```python
from build123d import *

# Parameters (mm, degrees)
CROQUIS1_R              = 1.5
SALIENTE_EXTRUIR1_DEPTH = 9
CROQUIS2_W              = 20
CROQUIS2_H              = 3.5
CORTAR_EXTRUIR1_DEPTH   = 18
REDONDEO1_R             = 3
CORTAR_EXTRUIR2_START   = -50
CORTAR_EXTRUIR2_DEPTH   = 50


# Read off the part's stored shape, not the designer's step: Cortar-Extruir2
with BuildPart() as part:
    # Croquis1 → Saliente-Extruir1 (new body)
    with BuildSketch(Plane(origin=(0, 0, 0), x_dir=(1, 0, 0), z_dir=(0, 1, 0))):
        Polygon((0, 0), (0, 10), (10, 16), (9, 10), (50, 10), (50, 0), align=None)
        with Locations(Location((25, 6, 0), (0, 0, 270))):
            Circle(CROQUIS1_R, mode=Mode.SUBTRACT)
    extrude(amount=SALIENTE_EXTRUIR1_DEPTH)

    # Croquis2 → Cortar-Extruir1 (cut)
    with BuildSketch(Plane(origin=(0, 9, 0), x_dir=(1, 0, 0), z_dir=(0, 1, 0))):
        with Locations((40, 8.25)):
            Rectangle(CROQUIS2_W, CROQUIS2_H)
    extrude(amount=-CORTAR_EXTRUIR1_DEPTH, mode=Mode.SUBTRACT)

    # Redondeo1
    redondeo1_edges = [part.edges().sort_by_distance(p)[0] for p in [
        (0, 4.5, -10),
        (30, 4.5, -10),
        (50, 4.5, -6.5),
    ]]
    fillet(redondeo1_edges, radius=REDONDEO1_R)

    # Cortar-Extruir2 outline → Cortar-Extruir2 (cut)
    with BuildSketch(Plane.ZY.offset(CORTAR_EXTRUIR2_START)):
        with BuildLine():
            ThreePointArc((-0.645847467, 9), (-0.162284879, 6.773055155), (0, 4.5))
            Line((0, 4.5), (0, 9))
            Line((0, 9), (-0.645847467, 9))
        make_face()
        with BuildLine():
            ThreePointArc((0, 4.5), (-0.162284879, 2.226944845), (-0.645847467, 0))
            Line((-0.645847467, 0), (0, 0))
            Line((0, 0), (0, 4.5))
        make_face()
    extrude(amount=CORTAR_EXTRUIR2_DEPTH, mode=Mode.SUBTRACT)


solid = part.part
```
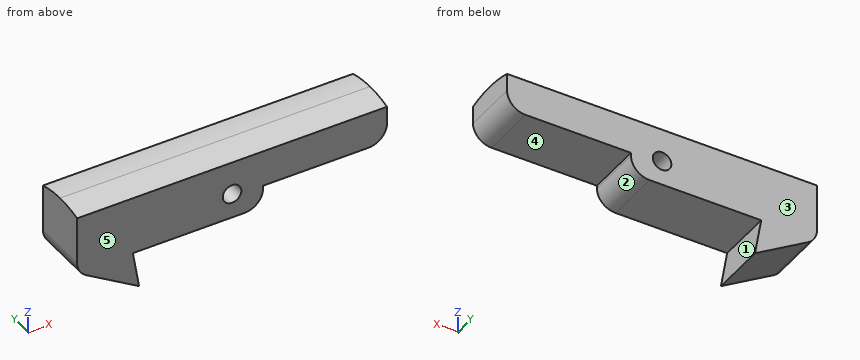
The listing builds one solid part. Answer for the finished solid, in the listing's coordinates (mm). Face numbers are marked on the shaded views. A direction names the side the tool comes from. Round coordinates to 2 decimals unless told otherwise and drop trailing zeros. Loops run counter-clockwise (first coordinate to the right, second up) from the corner with the lowest first, then second, coordinate; pieces in that order, holes last.
1) A cutting plane is placed at B-B on y = 2. Determine the outline of the cut face in (x, z).
Outcome:
outline: (0, -8.3) arc R3 ccw to (1.46, -10.87) - (10, -16) - (9, -10) - (27, -10) arc R3 ccw to (30, -7) - (30, -6.5) - (47, -6.5) arc R3 ccw to (50, -3.5) - (50, -0.2) - (0, -0.2) - close; hole circle Ø3 at (25, -6)
2) A cutting plane is placed at C-C on z = -6. Determine the outline of the cut face in (x, y), plus the area to 3 significant figures.
Outcome:
outline: (0, 0) - (23.5, 0) - (23.5, 9) - (0, 9) - close; (26.5, 0) - (48.66, 0) - (48.66, 9) - (26.5, 9) - close
area: 411 mm2
3) A cutting plane is placed at A-A on x = 25. Determine the outline of the cut face in (y, z), plus the area to 3 significant figures.
Outcome:
outline: (0, -10) - (9, -10) - (9, -7.5) - (0, -7.5) - close; (0, -4.5) - (9, -4.5) - (9, -0.65) arc R16 ccw to (0, -0.65) - close
area: 61.1 mm2
4) A cutting plane is placed at D-D on x = 4. Determine the outline of the cut face in (y, z), plus the area to 3 significant figures.
Outcome:
outline: (0, -12.4) - (9, -12.4) - (9, -0.65) arc R16 ccw to (0, -0.65) - close
area: 110 mm2
5) Consider line 1 (X direction, y = 5, z = -3.75); line 2 (X direction, y = 5.5, z = -6); line 3 (X direction, y = 0.5, z = -6.25). Determine where each line is inside the solid, lowest interval first.
Outcome:
line 1: x = 0 to 49.99
line 2: x = 0 to 23.5, 26.5 to 48.66
line 3: x = 0 to 23.52, 26.48 to 48.2
6) For the marked faces 4 and 5, determine the directions among +Z, -Z, +X, -X, +Y, -Y from which every point of the face is accessible in a straight line to the end or side of a thin tool.
Outcome:
face 4: -Z, +X, +Y, -Y
face 5: +Z, -Z, +X, -X, -Y
7) For a pull along Z with two mould halves and no side action, classify the marked faces 1, 2 and 3 as released by +Z, released by -Z, zero draft, split by the parting line, or undercut.
Outcome:
face 1: undercut
face 2: released by -Z
face 3: zero draft
8) Given P1, Ø1, axis at y = 1.5, z = -7.5, coming from the +X side, flat-ended and moving along its own axis, determine where the tip first touches the part or whether it passes through.
Outcome:
P1: stops at x = 30
